```python
from build123d import *

# Parameters (mm, degrees)
F1_DEPTH = 14.25
F2_R     = 1.25
F3_DEPTH = 10
F4_R     = 1.55
F5_DEPTH = 6


with BuildPart() as f1:
    # F0 (on Top) → F1 (new body)
    with BuildSketch(Plane.XY):
        Polygon((-1.917285, 2.603335), (-3.213197, -0.35875), (-1.295912, -2.962085), (1.917285, -2.603335), (3.213197, 0.35875), (1.295912, 2.962085), align=None)
    extrude(amount=F1_DEPTH)

    # F2 (on face) → F3 (cut)
    with BuildSketch(Plane(origin=(0, 0, 0), x_dir=(1, 0, 0), z_dir=(0, 0, -1))):
        Circle(F2_R)
    extrude(amount=-F3_DEPTH, mode=Mode.SUBTRACT)

    # F4 (on face) → F5 (join)
    with BuildSketch(Plane.XY.offset(14.25)):
        Circle(F4_R)
    extrude(amount=F5_DEPTH)


solid = f1.part
```
The listing builds one solid part. Answer for the finished solid, in the listing's coordinates (mm). A direction names the side the tool comes from. Coordinates: 2 decimals unless noted, no trailing zeros. Loops run counter-clockwise (first coordinate to the right, second up) from the corner with the lowest first, then second, coordinate; pieces in that order, holes last. Notation, with made-up numbers: (58, -39.5) -> (80, -39.5) arc R19 cw to (80, -2.5) -> close; hole circle Ø5 at (56, 70). An arc over 180 degrees is marked (long way). Return JSON: item names as keys, results as strings. Group by question number.
(1) A cutting plane is placed at D-D on y = 0.6. Write down the section's boundary in (x, z).
(2) Which of the six approach directions +Z, -Z, +X, -X, +Y, -Y give full straight-line access (tool end or side, diameter ignored) to faces 5 (the cylindrical face through (0.715, -1.375, 17.208)), 6 (the flat face through (-0.288, 2.785, 7.025))?
(3) A cutting plane is placed at A-A on z = 6.75. Write down the section's boundary in (x, y).
(4) A cutting plane is placed at C-C on x = 0.5. Write down the section's boundary in (y, z).
(5) Given pin 1 Ø3 at (y, z) = (-1.5, 2.5) entering from +X; pin 2 Ø2 at (y, z) = (2, 16.5) entering from +X, each flat-ended and moving along its own axis, determine where each tip first touches the part or whether it passes through.
(6) Determine the mould class of faces 1 (the cylindrical face through (-0.27, 1.22, 4.93)), 2 (the flat face through (0, 0, 10)), 3 (the flat face through (1, -1, 0)), 4 (the flat face through (0.288, -2.785, 7.025)) for opening direction X: released by +X, released by -X, zero draft, split by the parting line, or undercut.
(7) Find the intervals of material crossed by probe 1 along X at (y, z) = (0, 8); probe 2 along X at (y, z) = (0.5, 7.5); probe 3 along Z at (x, y) = (0, 0.2), in increasing order. Write a range as from..to.
(8) A cutting plane is placed at B-B on z = 17.5. Write down the section's boundary in (x, y), and give its area (3 significant figures).
The answers:
{
 "1": {"outline": "(-2.79, 0) -> (-1.1, 0) -> (-1.1, 10) -> (1.1, 10) -> (1.1, 0) -> (3.04, 0) -> (3.04, 14.25) -> (1.43, 14.25) -> (1.43, 20.25) -> (-1.43, 20.25) -> (-1.43, 14.25) -> (-2.79, 14.25) -> close"},
 "2": {"face 5": "+Z", "face 6": "+Z, -Z, -X, +Y"},
 "3": {"outline": "(-3.21, -0.36) -> (-1.3, -2.96) -> (1.92, -2.6) -> (3.21, 0.36) -> (1.3, 2.96) -> (-1.92, 2.6) -> close; hole circle Ø2.5 at (0, 0)"},
 "4": {"outline": "(-2.76, 0) -> (-1.15, 0) -> (-1.15, 10) -> (1.15, 10) -> (1.15, 0) -> (2.87, 0) -> (2.87, 14.25) -> (1.47, 14.25) -> (1.47, 20.25) -> (-1.47, 20.25) -> (-1.47, 14.25) -> (-2.76, 14.25) -> close"},
 "5": {"pin 1": "stops at x = 3.06", "pin 2": "stops at x = 1.18"},
 "6": {"face 1": "undercut", "face 2": "undercut", "face 3": "zero draft", "face 4": "released by +X"},
 "7": {"probe 1": "x = -3.06..-1.25, 1.25..3.06", "probe 2": "x = -2.84..-1.15, 1.15..3.11", "probe 3": "z = 10..20.25"},
 "8": {"outline": "circle Ø3.1 at (0, 0)", "area": "7.55 mm^2"}
}
